Autodesk Inventor part; units mm, degrees
ref_plane "YZ Plane" through (0, 0, 0) normal (1, 0, 0) x (0, 1, 0)
ref_plane "XZ Plane" through (0, 0, 0) normal (0, 1, 0) x (-1, 0, 0)
ref_plane "XY Plane" through (0, 0, 0) normal (0, 0, 1) x (1, 0, 0)
sketch "Sketch1" plane through (0, 0, 0) normal (0, 1, 0) x (-1, 0, 0)
  circle A0 centre (0, 0) radius 3.25
  circle A1 centre (0, 0) radius 4.5
  dimension "d0" = 6.5
  dimension "d1" = 9
extrude "Extrusion1" add sketch "Sketch1" along normal blind 3
extrude "Extrusion2" add sketch "Sketch1" along normal blind 1 contours A0
fillet "Fillet1" radius 1 1 edges at (4.5, 0, 0)
properties part number "button_cap"
CAD build for the part. Positions are in the model's coordinates, mm. A direction names the side the tool comes from. Give positions to 0.01 mm unless a question says otherwise; leave off trailing zeros. Order: outer loops, then holes, each group sorted by start corner. A loop starts at its lowest first (then second) coordinate and runs counter-clockwise, first axis right, second up. Notation, with made-up numbers: (-19, 85.5) -> (-13, 85.5) arc R8 cw to (-13, 100.5) -> close; hole circle Ø8 at (81.25, 54.5). An arc over 180 degrees is marked (long way). Return JSON: item names as keys, results as strings.
Q1. Flat gauge pins, fed straight in: pin 1 (5 mm diameter, centred on x = 0, z = 0, fed in from +Y); pin 2 (1 mm diameter, centred on y = 2, z = -2.5, fed in from -X); pin 3 (1.5 mm diameter, centred on x = 2.5, y = 2, fed in from -Z). Where does each tip first touch, or does it go through?
Working result:
{"pin 1": "y = 1", "pin 2": "x = -4.03", "pin 3": "z = -4.15"}
Q2. Which spindle directions (+Z, -Z, +X, -X, +Y, -Y) get a long thin tool onto all of the face, cutting with end or side? Do faces 1 (the face through (0.59, 1.99, -4.46)), 2 (the face through (0, 1, 0)). Say none if no direction does.
Working result:
{"face 1": "+Y, -Y", "face 2": "+Y"}
Q3. Saw through at C-C (z = 0). Write the cut outline in (x, y).
Working result:
{"outline": "(-4.5, 1) arc R1 ccw to (-3.5, 0) -> (3.5, 0) arc R1 ccw to (4.5, 1) -> (4.5, 3) -> (3.25, 3) -> (3.25, 1) -> (-3.25, 1) -> (-3.25, 3) -> (-4.5, 3) -> close"}
Q4. Saw through at B-B (y = 1.75). Write the cut outline in (x, z).
Working result:
{"outline": "circle Ø9 at (0, 0); hole circle Ø6.5 at (0, 0)"}
Q5. Saw through at A-A (x = 0). Write the cut outline in (y, z).
Working result:
{"outline": "(0, -3.5) arc R1 ccw to (1, -4.5) -> (3, -4.5) -> (3, -3.25) -> (1, -3.25) -> (1, 3.25) -> (3, 3.25) -> (3, 4.5) -> (1, 4.5) arc R1 ccw to (0, 3.5) -> close"}
Q6. Drill centre lines: line 1 (Z direction, x = 0, y = 2); line 2 (Y direction, x = 1, z = 0.75); line 3 (X direction, y = 2.4, z = 0.5). Where is each one in solid material? Low to high.
Working result:
{"line 1": "-4.5 to -3.25, 3.25 to 4.5", "line 2": "0 to 1", "line 3": "-4.47 to -3.21, 3.21 to 4.47"}
Q7. Saw through at D-D (y = 0.45). Write the cut outline in (x, z).
Working result:
{"outline": "circle Ø8.67 at (0, 0)"}
